Can you work these out from the model? Positions are in its coordinate system, mm. A direction names the side the tool comes from. Coordinates: 2 decimals unless noted, no trailing zeros. Write each loop counter-clockwise with the first axis right and the second up, starting at its lowest first coordinate (ties: lowest second). Pieces come first, ordered by that corner, then holes.
```python
from build123d import *

# Parameters (mm, degrees)
PAD_DEPTH = 10


with BuildPart() as part:
    # Sketch → Pad (new body)
    with BuildSketch(Plane.XY):
        with BuildLine():
            ThreePointArc((-7.827064, 6.656778), (0, -10.275), (7.827064, 6.656778))
            ThreePointArc((7.87625, 7.87625), (7.613377, 7.276125), (7.827064, 6.656778))
            Line((7.87625, 7.87625), (8.071323, 8.071323))
            ThreePointArc((9.392168, 8.019331), (8.743117, 8.33423), (8.071323, 8.071323))
            ThreePointArc((12.35, 0), (11.586971, 4.273712), (9.392168, 8.019331))
            Line((12.35, 0), (12.35, -24.275))
            Line((12.35, -24.275), (-12.35, -24.275))
            Line((-12.35, -24.275), (-12.35, 0))
            ThreePointArc((-9.392168, 8.019331), (-11.586971, 4.273712), (-12.35, 0))
            ThreePointArc((-8.071323, 8.071323), (-8.743117, 8.33423), (-9.392168, 8.019331))
            Line((-8.071323, 8.071323), (-7.87625, 7.87625))
            ThreePointArc((-7.827064, 6.656778), (-7.613377, 7.276125), (-7.87625, 7.87625))
        make_face()
    extrude(amount=PAD_DEPTH)


solid = part.part
```
1. If we section it at D-D, the plane y = -0.5: List the corners of the cut face in (x, z) for me.
2. Which directions (+Z, -Z, +X, -X, +Y, -Y) give clear straight access to the entire face, cutting with the end or side of a thin tool? Please do faces 4 (the face through (0, -11, 10)), 5 (the face through (7.614, 7.286, 4.93)).
3. If we section it at A-A, the plane y = -9: List the corners of the cut face in (x, z) for me, plus the area to 3 significant figures.
4. If we section it at C-C, the plane x = 0: List the corners of the cut face in (y, z) for me (3 decimals), plus the area to 3 significant figures.
5. We'd pull the mould along Y, two halves only. Please class faces 1 (the face through (0, -24.275, 5)), 2 (the face through (-11.566, 4.331, 4.93)), 3 (the face through (-7.613, 7.267, 4.93)): released by +Y, released by -Y, zero draft, split by the parting line, or undercut.
6. If I drill on L1, parallel to X at y = 3, z = 4; L2, parallel to X at y = -2, z = 6.5; L3, parallel to Y at x = -8, z = 1.75 (3 decimals), over which ranges is the centre line in solid material (lowest first)?
7. If we section it at B-B, the plane z = 7.75: List the corners of the cut face in (x, y) for me (3 decimals).
Answers:
1. outline: (-12.35, 0) - (-10.26, 0) - (-10.26, 10) - (-12.35, 10) - close; (10.26, 0) - (12.35, 0) - (12.35, 10) - (10.26, 10) - close
2. face 4: +Z, +X, -X, +Y, -Y
2. face 5: +Z, -Z
3. outline: (-12.35, 0) - (-4.96, 0) - (-4.96, 10) - (-12.35, 10) - close; (4.96, 0) - (12.35, 0) - (12.35, 10) - (4.96, 10) - close
3. area: 148 mm2
4. outline: (-24.275, 0) - (-10.275, 0) - (-10.275, 10) - (-24.275, 10) - close
4. area: 140 mm2
5. face 1: released by -Y
5. face 2: released by +Y
5. face 3: undercut
6. L1: x = -11.98 to -9.83, 9.83 to 11.98
6. L2: x = -12.35 to -10.08, 10.08 to 12.35
6. L3: y = -24.275 to -6.448, 6.448 to 8
7. outline: (-12.35, -24.275) - (12.35, -24.275) - (12.35, 0) arc R12.35 ccw to (9.392, 8.019) arc R0.9 ccw to (8.071, 8.071) - (7.876, 7.876) arc R0.9 ccw to (7.827, 6.657) arc R10.275 cw (long way) to (-7.827, 6.657) arc R0.9 ccw to (-7.876, 7.876) - (-8.071, 8.071) arc R0.9 ccw to (-9.392, 8.019) arc R12.35 ccw to (-12.35, 0) - close
